Could you check a few things on this model? Use its own coordinates, in mm. Face numbers are marked on the shaded views. A direction names the side the tool comes from. Give positions to 0.01 mm unless a question says otherwise; leave off trailing zeros. Write each loop counter-clockwise with the first axis right and the second up, starting at its lowest first coordinate (ties: lowest second). Pieces come first, ordered by that corner, then holes. Notation, with made-up numbers: (64, -13.75) - (86, -13.75) arc R26 ccw to (86, 17.25) - close; hole circle Ø9 at (74.5, 40). An arc over 180 degrees is marked (long way). Answer in a Markdown table with one row per item.
from build123d import *

# Parameters (mm, degrees)
SKETCH_1_R            = 1.65
EXTRUDE_241_DEPTH     = 1.6
EXTRUDE_START         = 1.6
SKETCH_2_W            = 42
SKETCH_2_H            = 40
EXTRUDE_307_DEPTH     = 6.4
CUT_EXTRUDE_START     = 1.6
SKETCH_3_R            = 3.5
CUT_EXTRUDE_391_DEPTH = 6.4


with BuildPart() as part:
    # 草图1 → Extrude 241 (new body)
    with BuildSketch(Plane.XY):
        Polygon((-22, -25), (22, -25), (25, -22), (25, 22), (22, 25), (-22, 25), (-25, 22), (-25, -22), align=None)
        with Locations((-15.25, -15.25)):
            Circle(SKETCH_1_R, mode=Mode.SUBTRACT)
        with Locations((-15.25, 15.25)):
            Circle(SKETCH_1_R, mode=Mode.SUBTRACT)
        with Locations((15.25, -15.25)):
            Circle(SKETCH_1_R, mode=Mode.SUBTRACT)
        with Locations((15.25, 15.25)):
            Circle(SKETCH_1_R, mode=Mode.SUBTRACT)
    extrude(amount=EXTRUDE_241_DEPTH)

    # 草图2 → Extrude 307 (add)
    with BuildSketch(Plane.XY.offset(EXTRUDE_START)):
        Rectangle(SKETCH_2_W, SKETCH_2_H)
    extrude(amount=EXTRUDE_307_DEPTH)

    # 草图3 → Cut-Extrude 391 (cut)
    with BuildSketch(Plane.XY.offset(CUT_EXTRUDE_START)):
        with Locations((-15.25, -15.25)):
            Circle(SKETCH_3_R)
        with Locations((-15.25, 15.25)):
            Circle(SKETCH_3_R)
        with Locations((15.25, -15.25)):
            Circle(SKETCH_3_R)
        with Locations((15.25, 15.25)):
            Circle(SKETCH_3_R)
    extrude(amount=CUT_EXTRUDE_391_DEPTH, mode=Mode.SUBTRACT)


solid = part.part
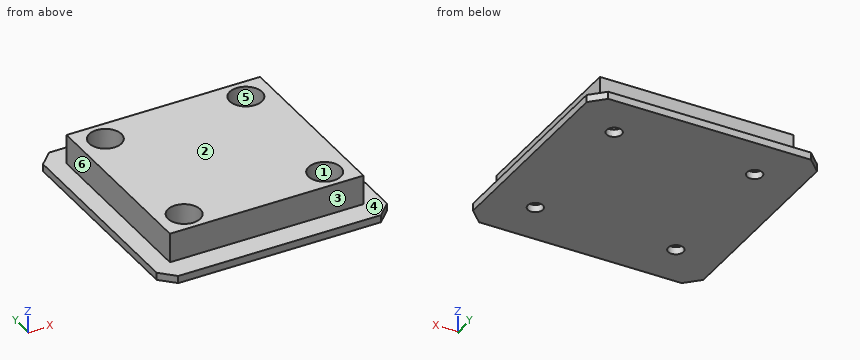
1) Will these pins go through, and if not, where does the flat tip stop? P1, Ø7.5, axis at x = -15, y = 14, coming from the +Z side; P2, Ø3, axis at y = 9, z = 4.5, coming from the +X side; P3, Ø3.5, axis at x = -15.5, y = -14, coming from the +Z side; P4, Ø1.9, axis at x = 9, z = 3.5, coming from the -Y side.
Check values:
| item | result |
|---|---|
| P1 | stops at z = 8 |
| P2 | stops at x = 21 |
| P3 | stops at z = 1.6 |
| P4 | stops at y = -20 |
2) We'd pull the mould along X, two halves only. Please class the marked faces 4, 5 and 6: +X half, -X half, draft (parallel to the pull), parting line (faces both ways), or undercut.
Check values:
| item | result |
|---|---|
| face 4 | draft |
| face 5 | undercut |
| face 6 | -X half |
3) Imagine slicing it at D-D (x = 2). List the corners of the cut face in (y, z) for me.
Check values:
| item | result |
|---|---|
| outline | (-25, 0) - (25, 0) - (25, 1.6) - (20, 1.6) - (20, 8) - (-20, 8) - (-20, 1.6) - (-25, 1.6) - close |
4) Imagine slicing it at B-B (z = 3.75). List the corners of the cut face in (x, y) for me, then the cut area to 3 significant figures.
Check values:
| item | result |
|---|---|
| outline | (-21, -20) - (21, -20) - (21, 20) - (-21, 20) - close; hole circle Ø7 at (-15.25, -15.25); hole circle Ø7 at (-15.25, 15.25); hole circle Ø7 at (15.25, -15.25); hole circle Ø7 at (15.25, 15.25) |
| area | 1,530 mm2 |
5) On a 3-axis mill with a long thin cutter (end or side, diameter ignored), from which of +Z, -Z, +X, -X, +Y, -Y can I reach the whole of each face in a straight line? I mean the marked faces 1, 2 and 3. Say none if no direction works.
Check values:
| item | result |
|---|---|
| face 1 | +Z |
| face 2 | +Z, +X, -X, +Y, -Y |
| face 3 | +Z, +X, -X, -Y |
6) Imagine slicing it at A-A (y = -15.25). List the corners of the cut face in (x, z) for me.
Check values:
| item | result |
|---|---|
| outline | (-25, 0) - (-16.9, 0) - (-16.9, 1.6) - (-18.75, 1.6) - (-18.75, 8) - (-21, 8) - (-21, 1.6) - (-25, 1.6) - close; (-13.6, 0) - (13.6, 0) - (13.6, 1.6) - (11.75, 1.6) - (11.75, 8) - (-11.75, 8) - (-11.75, 1.6) - (-13.6, 1.6) - close; (16.9, 0) - (25, 0) - (25, 1.6) - (21, 1.6) - (21, 8) - (18.75, 8) - (18.75, 1.6) - (16.9, 1.6) - close |
7) If I drill on line 1 (Y direction, x = -15.25, z = 0.8); line 2 (X direction, y = -12.5, z = 2.5); line 3 (X direction, y = -13.5, z = 1.75), over which ranges is the centre line in solid material (lowest first)?
Check values:
| item | result |
|---|---|
| line 1 | y = -25 to -16.9, -13.6 to 13.6, 16.9 to 25 |
| line 2 | x = -21 to -17.42, -13.08 to 13.08, 17.42 to 21 |
| line 3 | x = -21 to -18.28, -12.22 to 12.22, 18.28 to 21 |
8) Imagine slicing it at C-C (x = -15.25). List the corners of the cut face in (y, z) for me, then the cut area to 3 significant figures.
Check values:
| item | result |
|---|---|
| outline | (-25, 0) - (-16.9, 0) - (-16.9, 1.6) - (-18.75, 1.6) - (-18.75, 8) - (-20, 8) - (-20, 1.6) - (-25, 1.6) - close; (-13.6, 0) - (13.6, 0) - (13.6, 1.6) - (11.75, 1.6) - (11.75, 8) - (-11.75, 8) - (-11.75, 1.6) - (-13.6, 1.6) - close; (16.9, 0) - (25, 0) - (25, 1.6) - (20, 1.6) - (20, 8) - (18.75, 8) - (18.75, 1.6) - (16.9, 1.6) - close |
| area | 236 mm2 |
